Study the drawing (mm; zero at the part's minimum x, y, z) and answer. Round coordinates to 2 decimals unless told otherwise and drop trailing zeros. Write each loop counter-clockwise with the first axis right and the second up, starting at its lowest first coordinate (ties: lowest second). Pieces come first, ordered by that corner, then holes. Notation, with made-up numbers: (74.5, -25) - (105.5, -25) arc R21 cw to (105.5, 4) - close; hole circle Ø10 at (-24.75, -14.5). An arc over 180 degrees is marked (long way). Return JSON: item names as keys, results as strings. Group by question number.
(1) Section D-D, the plane y = 10.5 is taken. Write down the section's boundary in (x, z) (1 decimal).
(2) Determine the mould class of the marked faces 1, 2 and 3 for opening direction Y: +Y half, -Y half, draft (parallel to the pull), parting line (faces both ways), or undercut.
(3) Find the intervals of material crossed by line 1 along Y through (x, z) = (50.5, 78) (1 decimal); line 2 along Z through (x, y) = (13, 18) (1 decimal); line 3 along Y through (x, z) = (21, 23) (1 decimal), in increasing order. Write a range as [from, to].
(4) Each of these flat-tipped pins is pushed along its axis until it touches: pin 1 (8 mm diameter, centred on x = 25.5, y = 34, fed in from +Z); pin 2 (10 mm diameter, centred on x = 36.5, z = 26, fed in from -Y); pin 3 (6 mm diameter, centred on x = 46, y = 29.5, fed in from +Z). Where does it stop, or does it pass through?
(5) Section B-B, the plane x = 62 is taken. Write down the section's boundary in (y, z) (1 decimal).
(6) Section C-C, the plane z = 13 is taken. Write down the section's boundary in (x, y) (1 decimal), then the cut area to 3 significant figures.
(7) Section A-A, the plane y = 71 is taken. Write down the section's boundary in (x, z), then the cut area to 3 significant figures.
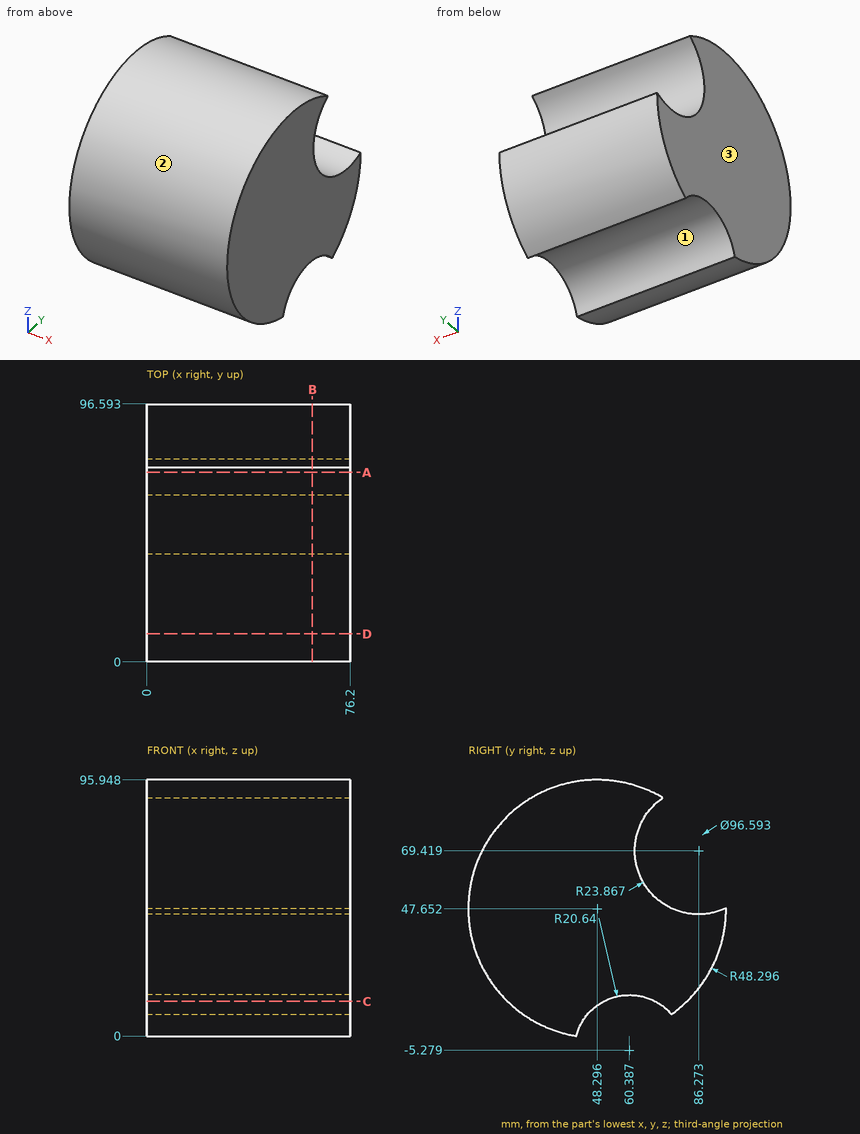
Working result:
{
 "1": {"outline": "(0, 17.6) - (76.2, 17.6) - (76.2, 77.7) - (0, 77.7) - close"},
 "2": {"face 1": "undercut", "face 2": "parting line", "face 3": "draft"},
 "3": {"line 1": "y = [10.7, 64]", "line 2": "z = [10, 85.3]", "line 3": "y = [6.8, 89.8]"},
 "4": {"pin 1": "stops at z = 94.84", "pin 2": "stops at y = 2.96", "pin 3": "stops at z = 93.29"},
 "5": {"outline": "(40.4, 0) arc R20.6 cw to (76.1, 8.1) arc R48.3 ccw to (96.6, 47.9) arc R23.9 cw to (72.9, 89.2) arc R48.3 ccw (long way) to start"},
 "6": {"outline": "(0, 14.7) - (76.2, 14.7) - (76.2, 50.8) - (0, 50.8) - close; (0, 70) - (76.2, 70) - (76.2, 81.9) - (0, 81.9) - close", "area": "3,670 mm^2"},
 "7": {"outline": "(0, 12.42) - (76.2, 12.42) - (76.2, 51.08) - (0, 51.08) - close; (0, 87.76) - (76.2, 87.76) - (76.2, 90.28) - (0, 90.28) - close", "area": "3,140 mm^2"}
}
